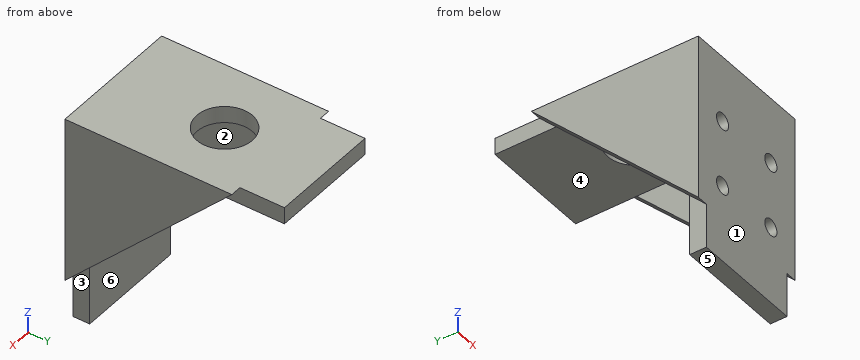
```python
from build123d import *

# Parameters (mm, degrees)
EXTRUDE_1_DEPTH     = 20
SKETCH_3_R          = 1.5
CUT_EXTRUDE_1_DEPTH = 56.398555938
SKETCH_5_R          = 5
CUT_EXTRUDE_3_DEPTH = 56.398555938
EXTRUDE_2_DEPTH     = 2
EXTRUDE_3_DEPTH     = 2


with BuildPart() as part:
    # 草图1 → 凸台-拉伸1 (new body)
    with BuildSketch(Plane(origin=(0, 0, 0), x_dir=(0, 0, -1), z_dir=(1, 0, 0))):
        Polygon((0, 0), (0, 38), (3, 38), (3, 3), (38, 3), (38, 0), align=None)
    extrude(amount=EXTRUDE_1_DEPTH)

    # 草图3 → 切除-拉伸1 (cut, through all)
    with BuildSketch(Plane(origin=(0, 3, 0), x_dir=(1, 0, 0), z_dir=(0, 1, 0))):
        with Locations(Location((16, 12, 0), (0, 0, 270))):
            Circle(SKETCH_3_R)
        with Locations(Location((4, 12, 0), (0, 0, 270))):
            Circle(SKETCH_3_R)
        with Locations(Location((4, 24, 0), (0, 0, 270))):
            Circle(SKETCH_3_R)
        with Locations(Location((16, 24, 0), (0, 0, 270))):
            Circle(SKETCH_3_R)
    extrude(amount=-CUT_EXTRUDE_1_DEPTH, mode=Mode.SUBTRACT)

    # 草图5 → 切除-拉伸3 (cut, through all)
    with BuildSketch(Plane(origin=(0, 0, -3), x_dir=(-1, 0, 0), z_dir=(0, 0, -1))):
        with Locations((-10, 20)):
            Circle(SKETCH_5_R)
    extrude(amount=-CUT_EXTRUDE_3_DEPTH, mode=Mode.SUBTRACT)

    # 草图6 → 凸台-拉伸2 (add)
    with BuildSketch(Plane.ZY):
        Polygon((0, 0), (0, 30), (-30, 0), align=None)
    extrude(amount=EXTRUDE_2_DEPTH)

    # 草图7 → 凸台-拉伸3 (add)
    with BuildSketch(Plane(origin=(20, 0, 0), x_dir=(0, 0, -1), z_dir=(1, 0, 0))):
        Polygon((0, 0), (0, 30), (30, 0), align=None)
    extrude(amount=EXTRUDE_3_DEPTH)


solid = part.part
```
CAD build for the part. Positions are in the model's coordinates, mm. Face numbers are marked on the shaded views. A direction names the side the tool comes from. Coordinates: 2 decimals unless noted, no trailing zeros. Order: outer loops, then holes, each group sorted by start corner. A loop starts at its lowest first (then second) coordinate and runs counter-clockwise, first axis right, second up. Notation, with made-up numbers: (72, 37) - (109, 37) arc R37 ccw to (109, 73) - close; hole circle Ø10 at (55, -33). An arc over 180 degrees is marked (long way). Answer in a Markdown table with one row per item.
1. Slice it at D-D, the plane x = 16. List the corners of the cut face in (y, z).
Answer:
| item | result |
|---|---|
| outline | (0, -38) - (3, -38) - (3, -25.5) - (0, -25.5) - close; (0, -22.5) - (3, -22.5) - (3, -13.5) - (0, -13.5) - close; (0, -10.5) - (3, -10.5) - (3, -3) - (38, -3) - (38, 0) - (0, 0) - close |
2. Slice it at B-B, the plane z = -12. List the corners of the cut face in (x, y), then the cut area to 3 significant figures.
Answer:
| item | result |
|---|---|
| outline | (-2, 0) - (2.5, 0) - (2.5, 3) - (0, 3) - (0, 18) - (-2, 18) - close; (5.5, 0) - (14.5, 0) - (14.5, 3) - (5.5, 3) - close; (17.5, 0) - (22, 0) - (22, 18) - (20, 18) - (20, 3) - (17.5, 3) - close |
| area | 114 mm² |
3. Flat gauge pins, fed straight in: P1, Ø2.5, axis at y = 31, z = -2, coming from the -X side; P2, Ø2, axis at x = 18.5, y = 20.5, coming from the -Z side; P3, Ø4, axis at x = 15, z = -9.5, coming from the +Y side. Where does each tip first touch, or does it go through?
Answer:
| item | result |
|---|---|
| P1 | x = 0 |
| P2 | z = -3 |
| P3 | y = 3 |
4. Slice it at A-A, the plane x = 13. List the corners of the cut face in (y, z).
Answer:
| item | result |
|---|---|
| outline | (0, -38) - (3, -38) - (3, -3) - (16, -3) - (16, 0) - (0, 0) - close; (24, -3) - (38, -3) - (38, 0) - (24, 0) - close |
5. 3-axis set-ups, long thin cutter, end or side, ignore diameter. For the marked faces 5 and 6: which of +Z, -Z, +X, -X, +Y, -Y reach the whole face in a straight line?
Answer:
| item | result |
|---|---|
| face 5 | -Z, +X, -X, +Y, -Y |
| face 6 | -Z, +Y |
6. Drill centre lines: L1, parallel to X at y = 2, z = -24; L2, parallel to Y at x = 10, z = -2.3; L3, parallel to X at y = 15, z = -14.5. Where is each one in solid material? Low to high. Write a range as from..to.
Answer:
| item | result |
|---|---|
| L1 | -2..2.5, 5.5..14.5, 17.5..22 |
| L2 | 0..15, 25..38 |
| L3 | -2..0, 20..22 |
7. Slice it at C-C, the plane y = 20. List the corners of the cut face in (x, z), then the cut area to 3 significant figures.
Answer:
| item | result |
|---|---|
| outline | (-2, -10) - (0, -10) - (0, -3) - (5, -3) - (5, 0) - (-2, 0) - close; (15, -3) - (20, -3) - (20, -10) - (22, -10) - (22, 0) - (15, 0) - close |
| area | 70.0 mm² |
8. Pull direction X, two halves, no side cores. Call the marked faces 1, 2, 3 and 4: +X half, -X half, draft (parallel to the pull), parting line (faces both ways), or undercut.
Answer:
| item | result |
|---|---|
| face 1 | draft |
| face 2 | undercut |
| face 3 | +X half |
| face 4 | undercut |
